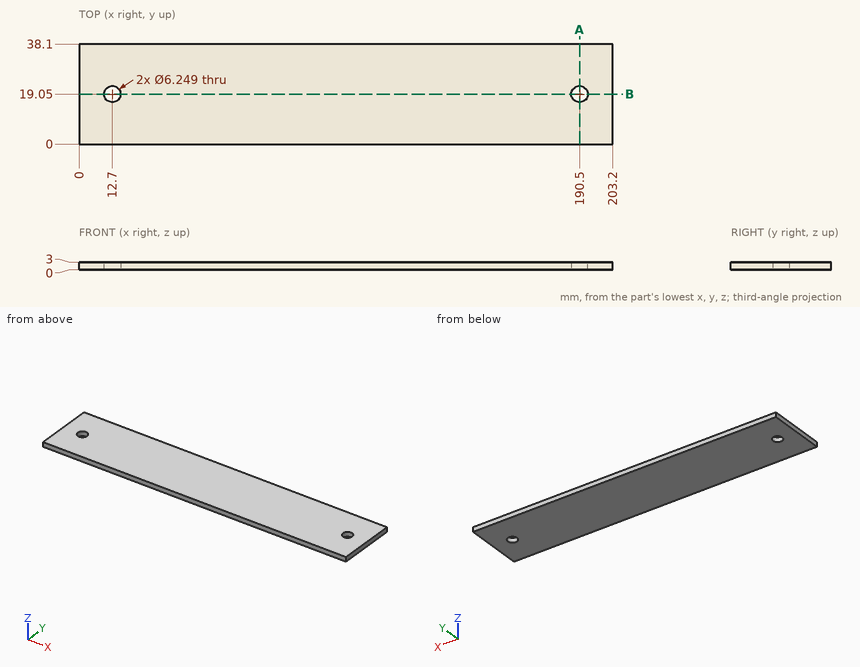
Drawing for the job (mm, zero at the part's lowest x, y, z). Coordinates: 2 decimals unless noted, no trailing zeros. Loops run counter-clockwise (first coordinate to the right, second up) from the corner with the lowest first, then second, coordinate; pieces in that order, holes last. Notation, with made-up numbers: (-22, -14) - (-2, -14) arc R12 cw to (-2, -9) - close; hole circle Ø3 at (17, 24). An arc over 180 degrees is marked (long way). Return JSON: item names as keys, results as strings.
1. Probe L1, parallel to X at y = 19.05, z = 1.15; L2, parallel to Y at x = 190.5, z = 1; L3, parallel to X at y = 20.5, z = 1.25. List the from-to ranges inside material, lowest first. Write a range as from..to.
Result:
{"L1": "x = 0..9.58, 15.82..187.38, 193.62..203.2", "L2": "y = 0..15.93, 22.17..38.1", "L3": "x = 0..9.93, 15.47..187.73, 193.27..203.2"}
2. Band-saw the part on B-B (y = 19.05). Give the cut face in (x, z).
Result:
{"outline": "(0, 0) - (9.58, 0) - (9.58, 3) - (0, 3) - close; (15.82, 0) - (187.38, 0) - (187.38, 3) - (15.82, 3) - close; (193.62, 0) - (203.2, 0) - (203.2, 3) - (193.62, 3) - close"}
3. Band-saw the part on A-A (x = 190.5). Give the cut face in (y, z).
Result:
{"outline": "(0, 0) - (15.93, 0) - (15.93, 3) - (0, 3) - close; (22.17, 0) - (38.1, 0) - (38.1, 3) - (22.17, 3) - close"}
